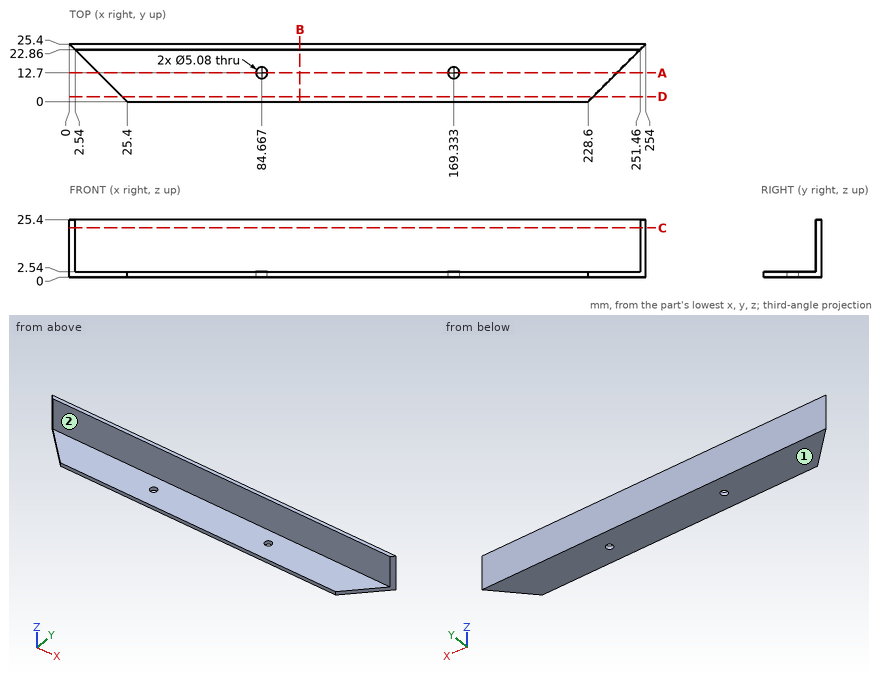
Answer from the drawing. Dimensions are ordinates in mm from the lowest x, y and z of the part. A direction names the side the tool comes from. Round coordinates to 2 decimals unless told otherwise and drop trailing zeros. Loops run counter-clockwise (first coordinate to the right, second up) from the corner with the lowest first, then second, coordinate; pieces in that order, holes last. Notation, with made-up numbers: (3.25, 42) - (7.25, 42) arc R22 ccw to (7.25, 80) - close; hole circle Ø7 at (38, 43.25). An arc over 180 degrees is marked (long way). Return JSON: item names as keys, results as strings. Group by question number.
1. Consider probe 1 along Y at (x, z) = (85, 2.5); probe 2 along X at (y, z) = (13, 2.25) (1 decimal); probe 3 along Y at (x, z) = (129.5, 7.5). Determine where each line is inside the solid, lowest interval first.
2. The part is cut by section A-A on y = 12.7. Determine the outline of the cut face in (x, z), then the cut area to 3 significant figures.
3. Each of these flat-tipped pins is pushed along its axis until it touches: P1, Ø6.5, axis at x = 84.67, y = 12.7, coming from the +Z side; P2, Ø10, axis at y = 12.5, z = 6.5, coming from the -X side; P3, Ø3, axis at x = 169.33, y = 12.7, coming from the -Z side. Where does it stop, or does it pass through?
4. The part is cut by section D-D on y = 2.25. Determine the outline of the cut face in (x, z).
5. Which of the six approach directions +Z, -Z, +X, -X, +Y, -Y give full straight-line access (tool end or side, diameter ignored) to the marked faces 1 and 2?
6. The part is cut by section B-B on x = 101.5. Determine the outline of the cut face in (y, z), then the cut area to 3 significant figures.
7. The part is cut by section C-C on z = 21.75. Determine the outline of the cut face in (x, y).
Resolved:
{
 "1": {"probe 1": "y = 0 to 10.18, 15.22 to 25.4", "probe 2": "x = 12.4 to 82.1, 87.2 to 166.8, 171.9 to 241.6", "probe 3": "y = 22.86 to 25.4"},
 "2": {"outline": "(12.7, 0) - (82.13, 0) - (82.13, 2.54) - (12.7, 2.54) - close; (87.21, 0) - (166.79, 0) - (166.79, 2.54) - (87.21, 2.54) - close; (171.87, 0) - (241.3, 0) - (241.3, 2.54) - (171.87, 2.54) - close", "area": "555 mm²"},
 "3": {"P1": "stops at z = 2.54", "P2": "stops at x = 9.85", "P3": "passes through"},
 "4": {"outline": "(23.15, 0) - (230.85, 0) - (230.85, 2.54) - (23.15, 2.54) - close"},
 "5": {"face 1": "-Z, +X, -X, +Y, -Y", "face 2": "+Z, +X, -X, -Y"},
 "6": {"outline": "(0, 0) - (25.4, 0) - (25.4, 25.4) - (22.86, 25.4) - (22.86, 2.54) - (0, 2.54) - close", "area": "123 mm²"},
 "7": {"outline": "(0, 25.4) - (2.54, 22.86) - (251.46, 22.86) - (254, 25.4) - close"}
}
